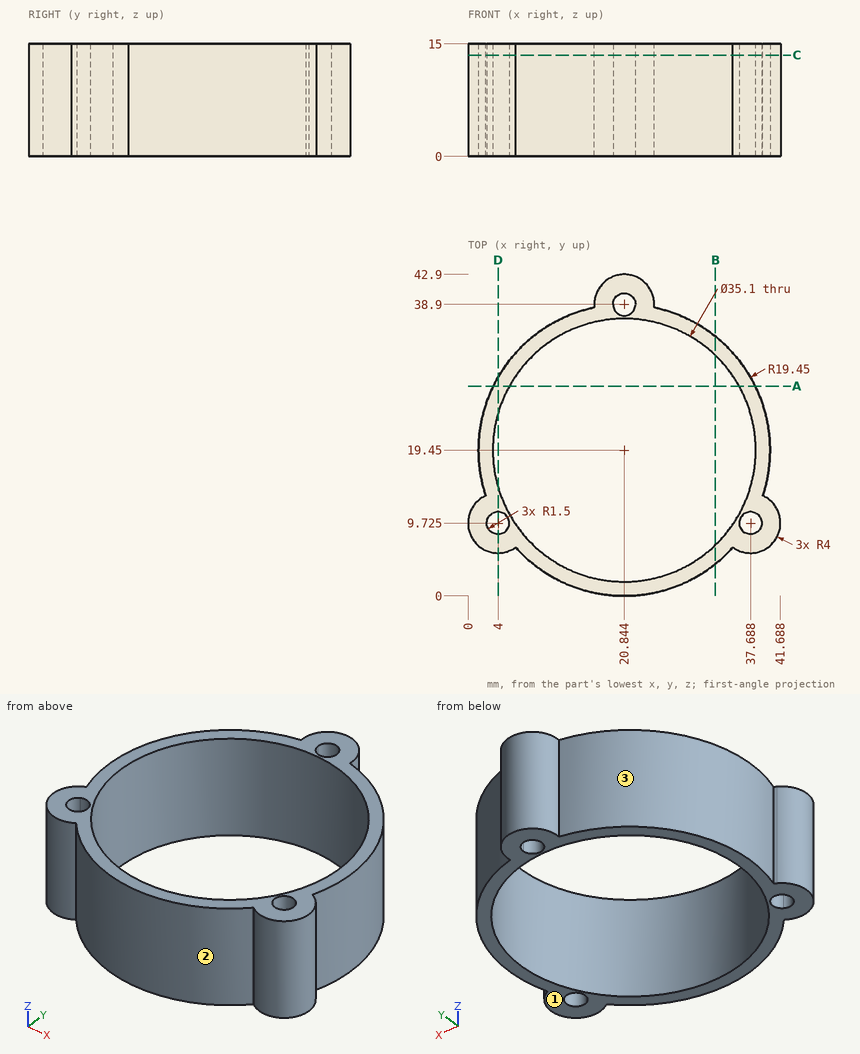
Geometry check sheet. Reference: drawing and pictorial views, mm from the part's lowest x, y, z. Give positions to 0.01 mm unless a question says otherwise; leave off trailing zeros. Order: outer loops, then holes, each group sorted by start corner. A loop starts at its lowest first (then second) coordinate and runs counter-clockwise, first axis right, second up. Notation, with made-up numbers: M -16,53 L -3,53 A8 cw -3,58 Z; hole C 0.5,34.5 d11. An arc over 180 degrees is marked long. Answer in a Markdown table with one row per item. Add a question column.
Q1. Release check for a two-part mould opening along Y. For the marked faces 1, 2 and 3 record: released by +Y, released by -Y, zero draft, split by the parting line, or undercut.
Q2. Sectioned sample at B-B, the plane x = 33. Record the boundary of the cut face in (y, z).
Q3. Thickness scan on L1, parallel to Y at x = 20.5, z = 11.25 (1 decimal); L2, parallel to X at y = 17.5, z = 1.75 (1 decimal); L3, parallel to X at y = 17, z = 2.75. Record the ranges inside material, lowest first.
Q4. Sectioned sample at D-D, the plane x = 4. Record the boundary of the cut face in (y, z) (1 decimal), and give its area (3 significant figures).
Q5. Sectioned sample at C-C, the plane z = 13.5. Count the separate pieces of the cut face and the enclosed holes in it.
Q6. Gauge pin test, flat ends, axial feed: pin 1 Ø1 at (y, z) = (4.5, 2.5) entering from -X (1 decimal); pin 2 Ø4 at (x, z) = (17, 9) entering from +Y; pin 3 Ø3 at (y, z) = (16, 9.5) entering from -X; pin 4 Ø21 at (x, y) = (20.84, 19.45) entering from +Z. Record the tip position at first contact, or that the pin passes through.
Q7. Sectioned sample at A-A, the plane y = 28. Record the boundary of the cut face in (x, z) (1 decimal).
Verdict:
| question | item | result |
|---|---|---|
| 1 | face 1 | zero draft |
| 1 | face 2 | released by -Y |
| 1 | face 3 | undercut |
| 2 | outline | M 4.27,0 L 6.79,0 L 6.79,15 L 4.27,15 Z; M 32.11,0 L 34.63,0 L 34.63,15 L 32.11,15 Z |
| 3 | L1 | 0 to 1.9, 37 to 37.4, 40.4 to 42.9 |
| 3 | L2 | 1.5 to 3.4, 38.3 to 40.2 |
| 3 | L3 | 1.55 to 3.47, 38.22 to 40.14 |
| 4 | outline | M 5.7,0 L 8.2,0 L 8.2,15 L 5.7,15 Z; M 11.2,0 L 14.5,0 L 14.5,15 L 11.2,15 Z; M 24.4,0 L 29.2,0 L 29.2,15 L 24.4,15 Z |
| 4 | area | 159 mm² |
| 5 | separate pieces | 1 |
| 5 | enclosed holes | 4 |
| 6 | pin 1 | x = 7.8 |
| 6 | pin 2 | y = 42.45 |
| 6 | pin 3 | x = 1.49 |
| 6 | pin 4 | through |
| 7 | outline | M 3.4,0 L 5.5,0 L 5.5,15 L 3.4,15 Z; M 36.2,0 L 38.3,0 L 38.3,15 L 36.2,15 Z |
